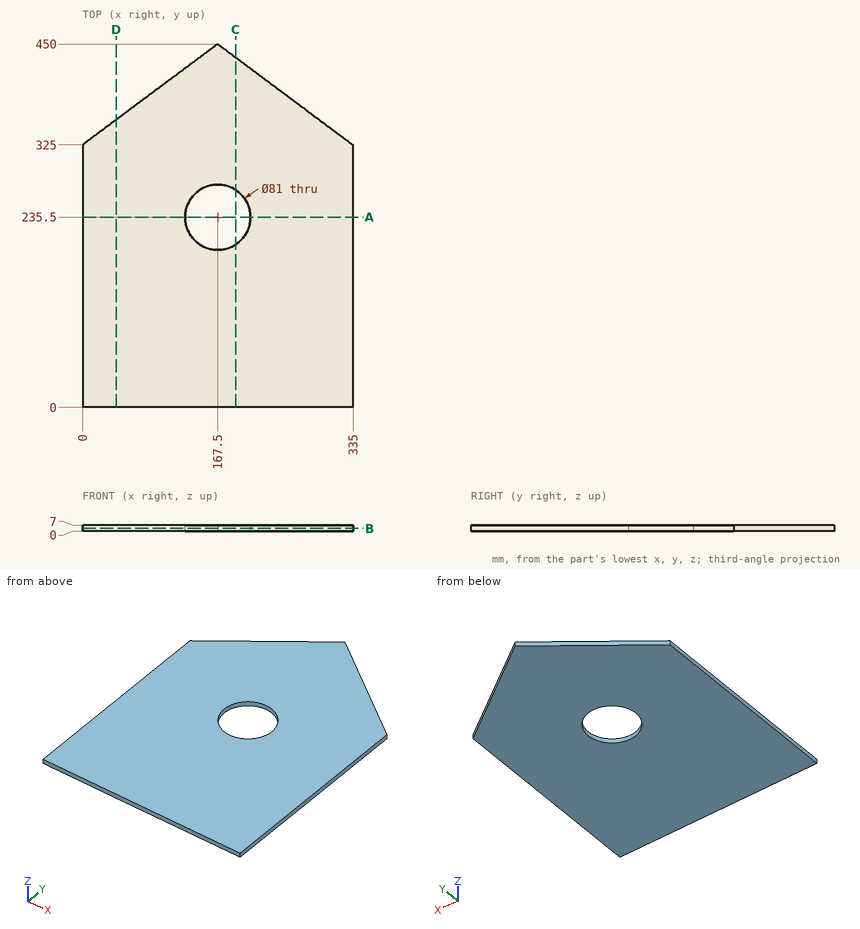
Study the drawing (mm; zero at the part's minimum x, y, z) and answer. Round coordinates to 2 decimals unless told otherwise and drop trailing zeros. Order: outer loops, then holes, each group sorted by start corner. A loop starts at its lowest first (then second) coordinate and runs counter-clockwise, first axis right, second up. Notation, with made-up numbers: (88, 78) - (128, 78) arc R16 ccw to (128, 109) - close; hole circle Ø7 at (-19.5, 65.5). An arc over 180 degrees is marked (long way). Use one line per item in the form item = value. Start each with the question number.
(1) Find the intervals of material crossed by line 1 along Y through (x, z) = (167.5, 3.5); line 2 along X through (y, z) = (235.5, 5); line 3 along X through (y, z) = (233.5, 6.75), in increasing order. Write a range as from..to.
(2) Flat-ended cylindrical pins translate along their axes: pin 1 Ø1 at (x, z) = (286.5, 4.5) entering from -Y; pin 2 Ø2 at (y, z) = (393, 3) entering from -X. Find the tip coordinate at first contact, or state that the pin passes through.
(3) The part is cut by section D-D (x = 41.5). Give the vertices of the cut face in (y, z), then the cut area to 3 significant figures.
(4) The part is cut by section C-C (x = 189.5). Give the vertices of the cut face in (y, z).
(5) The part is cut by section A-A (y = 235.5). Give the vertices of the cut face in (x, z).
(6) The part is cut by section B-B (z = 3.5). Give the vertices of the cut face in (x, y), then the cut area to 3 significant figures.
Checked values:
q1.line_1 = 0..195, 276..450
q1.line_2 = 0..127, 208..335
q1.line_3 = 0..127.05, 207.95..335
q2.pin_1 = 0
q2.pin_2 = 89.78
q3.outline = (0, 0) - (355.97, 0) - (355.97, 7) - (0, 7) - close
q3.area = 2,490 mm^2
q4.outline = (0, 0) - (201.5, 0) - (201.5, 7) - (0, 7) - close; (269.5, 0) - (433.58, 0) - (433.58, 7) - (269.5, 7) - close
q5.outline = (0, 0) - (127, 0) - (127, 7) - (0, 7) - close; (208, 0) - (335, 0) - (335, 7) - (208, 7) - close
q6.outline = (0, 0) - (335, 0) - (335, 325) - (167.5, 450) - (0, 325) - close; hole circle Ø81 at (167.5, 235.5)
q6.area = 125,000 mm^2
